Geometry check sheet. Reference: drawing and pictorial views, mm from the part's lowest x, y, z. A direction names the side the tool comes from. Give positions to 0.01 mm unless a question says otherwise; leave off trailing zeros. Loops run counter-clockwise (first coordinate to the right, second up) from the corner with the lowest first, then second, coordinate; pieces in that order, holes last. Notation, with made-up numbers: (76, 55.25) - (133, 55.25) arc R20 cw to (133, 84.25) - close; hole circle Ø5 at (16, 79). An arc over 180 degrees is marked (long way). Answer in a Markdown table with one row per item. Add a question column.
(1) Sectioned sample at D-D on y = 4.5. Enter the section's corners in (x, z).
(2) Set-up check for the marked faces 1, 2 and 3: record each of +Z, -Z, +X, -X, +Y, -Y from which the full face is reachable in a straight line by a thin tool's end or side.
(3) Sectioned sample at C-C on z = 40. Enter the section's corners in (x, y), then the cut area to 3 significant figures.
(4) Sectioned sample at A-A on y = 25. Enter the section's corners in (x, z).
(5) Sectioned sample at B-B on x = 75. Enter the section's corners in (y, z), then the cut area to 3 significant figures.
(6) Draft check along X on the marked faces 4, 5, 6 and 7. Enter one of: released by +X, released by -X, zero draft, split by the parting line, or undercut.
(7) Thickness scan on L1, parallel to Z at x = 75, y = 2.5; L2, parallel to X at y = 25, z = 29; L3, parallel to Y at x = 6, z = 22.5. Record the ranges inside material, lowest first.
(8) Go/stop test with flat-tipped pins: P1, Ø5, axis at y = 28.5, z = 15, coming from the +X side; P2, Ø6, axis at x = 5, z = 10, coming from the +Y side; P3, Ø2, axis at y = 17, z = 8.5, coming from the -X side. Record where each tip stops, or that it passes through.
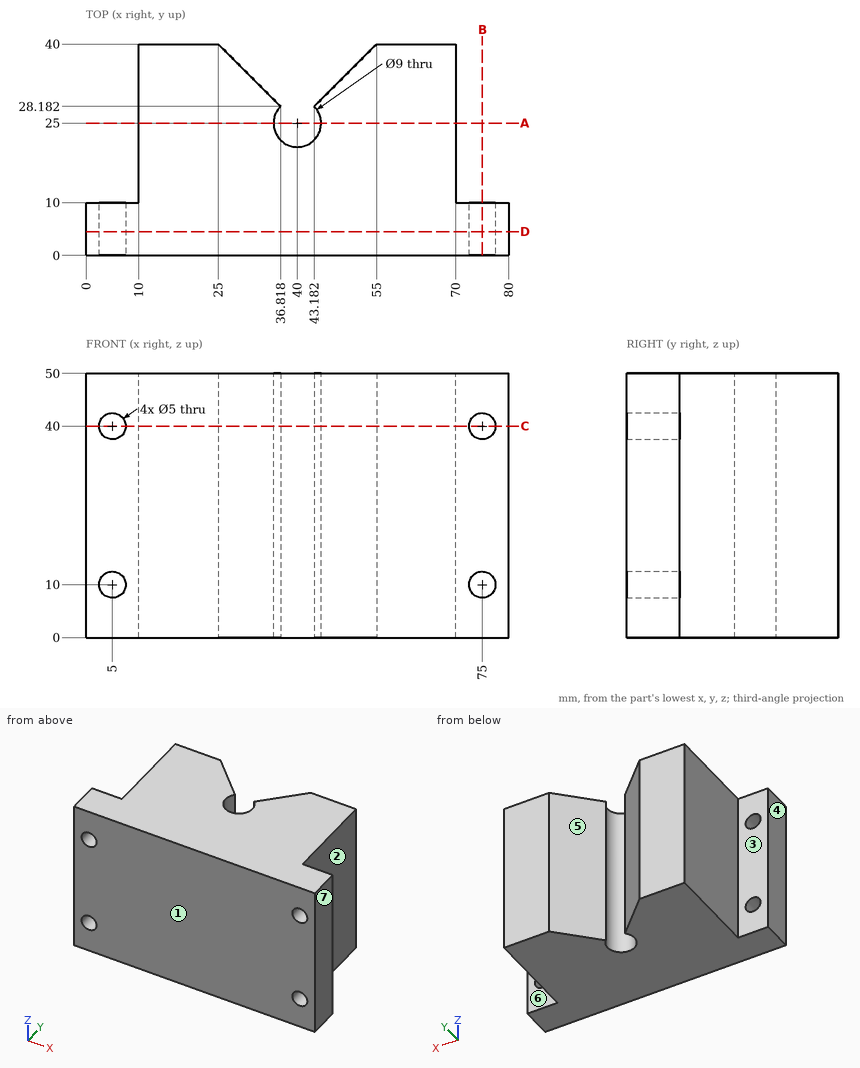
Reply:
| question | item | result |
|---|---|---|
| 1 | outline | (0, 0) - (80, 0) - (80, 50) - (0, 50) - close; hole circle Ø5 at (5, 10); hole circle Ø5 at (5, 40); hole circle Ø5 at (75, 10); hole circle Ø5 at (75, 40) |
| 2 | face 1 | +Z, -Z, +X, -X, -Y |
| 2 | face 2 | +Z, -Z, +X, +Y |
| 2 | face 3 | +Z, -Z, -X, +Y |
| 3 | outline | (0, 0) - (2.5, 0) - (2.5, 10) - (0, 10) - close; (7.5, 0) - (72.5, 0) - (72.5, 10) - (70, 10) - (70, 40) - (55, 40) - (43.18, 28.18) arc R4.5 cw (long way) to (36.82, 28.18) - (25, 40) - (10, 40) - (10, 10) - (7.5, 10) - close; (77.5, 0) - (80, 0) - (80, 10) - (77.5, 10) - close |
| 3 | area | 2,230 mm^2 |
| 4 | outline | (10, 0) - (35.5, 0) - (35.5, 50) - (10, 50) - close; (44.5, 0) - (70, 0) - (70, 50) - (44.5, 50) - close |
| 5 | outline | (0, 0) - (10, 0) - (10, 7.5) - (0, 7.5) - close; (0, 12.5) - (10, 12.5) - (10, 37.5) - (0, 37.5) - close; (0, 42.5) - (10, 42.5) - (10, 50) - (0, 50) - close |
| 5 | area | 400 mm^2 |
| 6 | face 4 | released by -X |
| 6 | face 5 | undercut |
| 6 | face 6 | zero draft |
| 6 | face 7 | released by +X |
| 7 | L1 | 0 to 7.5, 12.5 to 37.5, 42.5 to 50 |
| 7 | L2 | 10 to 35.5, 44.5 to 70 |
| 7 | L3 | 0 to 10 |
| 8 | P1 | x = 70 |
| 8 | P2 | y = 10 |
| 8 | P3 | x = 10 |
